```python
from build123d import *

# Parameters (mm, degrees)
SKETCH1_R           = 5.078298903
BOSS_EXTRUDE1_DEPTH = 3.175
SKETCH2_R           = 6.35
BOSS_EXTRUDE2_DEPTH = 50.8


with BuildPart() as part:
    # Sketch1 → Boss-Extrude1 (new body)
    with BuildSketch(Plane(origin=(0, 0, 0), x_dir=(1, 0, 0), z_dir=(0, 1, 0))):
        Polygon((-55.44099562, -40.268516884), (-128.460753109, 73.100956593), (-105.319843222, 83.572742001), (-32.300085734, -29.796731476), align=None)
        with Locations((-109.811555345, 67.600325735)):
            Circle(SKETCH1_R, mode=Mode.SUBTRACT)
    extrude(amount=BOSS_EXTRUDE1_DEPTH)

    # Sketch2 → Boss-Extrude2 (add)
    with BuildSketch(Plane(origin=(0, 3.175, 0), x_dir=(1, 0, 0), z_dir=(0, 1, 0))):
        with Locations((-50.696094851, -24.181527026)):
            Circle(SKETCH2_R)
    extrude(amount=BOSS_EXTRUDE2_DEPTH)


solid = part.part
```
Source: CAD feature listing. Evaluate the final solid. Frame: model axes, mm. A direction names the side the tool comes from. Give positions to 0.01 mm unless a question says otherwise; leave off trailing zeros. Loops run counter-clockwise (first coordinate to the right, second up) from the corner with the lowest first, then second, coordinate; pieces in that order, holes last. Notation, with made-up numbers: (-9.5, 73.25) -> (47.5, 73.25) arc R29 cw to (47.5, 98.25) -> close; hole circle Ø3 at (87, -38.5). An arc over 180 degrees is marked (long way). Put each result on its own line as item: value. Start each with the question number.
1) Cut plane D-D (y = 41.5). Return loops of the section in (x, z).
2) Material intervals for probe 1 along Y at (x, z) = (-97, -27.5) (3 decimals); probe 2 along Z at (x, y) = (-46, 46.5); probe 3 along Z at (x, y) = (-46.5, 36), sorted ascending.
3) Contact query for a flat-ended pin moving along its axis: P1, Ø1, axis at x = -50.5, y = 16, coming from the +Z side. Output: stop coordinate, or through.
4) Cut plane C-C (z = -24.5). Return loops of the section in (x, y) (3 decimals), then the cut area to 3 significant figures.
5) Draft query along Z for faces 1 (the face through (-80, 0, -17)), 2 (the face through (-113.84, 1.57, -64.51)), 3 (the face through (-43.71, 1.57, 34.96)). Return one class per face: released by +Z, released by -Z, zero draft, split by the parting line, or undercut.
6) Reachability of faces 4 (the face through (-69.32, 1.57, -27.68)), 5 (the face through (-57.04, 28.22, 23.9)) from +Z, -Z, +X, -X, +Y, -Y: full face, straight path, thin tool, end or side. Return the list, or none.
7) Cut plane A-A (x = -113.5). Return loops of the section in (y, z) (3 decimals), then the cut area to 3 significant figures.
8) Cut plane B-B (x = -53). Return loops of the section in (y, z) (3 decimals), then the cut area to 3 significant figures.
Results are:
1. outline: circle Ø12.7 at (-50.7, 24.18)
2. probe 1: y = 0 to 3.175
2. probe 2: z = 19.91 to 28.46
2. probe 3: z = 19.42 to 28.95
3. P1: stops at z = 30.53
4. outline: (-97.158, 0) -> (-67.272, 0) -> (-67.272, 3.175) -> (-97.158, 3.175) -> close
4. area: 94.9 mm2
5. face 1: zero draft
5. face 2: undercut
5. face 3: released by +Z
6. face 4: -Z, +X, +Y, -Y
6. face 5: +Y
7. outline: (0, -79.871) -> (3.175, -79.871) -> (3.175, -71.091) -> (0, -71.091) -> close; (0, -64.11) -> (3.175, -64.11) -> (3.175, -49.873) -> (0, -49.873) -> close
7. area: 73.1 mm2
8. outline: (0, -2.342) -> (3.175, -2.342) -> (3.175, 18.264) -> (53.975, 18.264) -> (53.975, 30.099) -> (3.175, 30.099) -> (3.175, 39.164) -> (0, 39.164) -> close
8. area: 733 mm2
